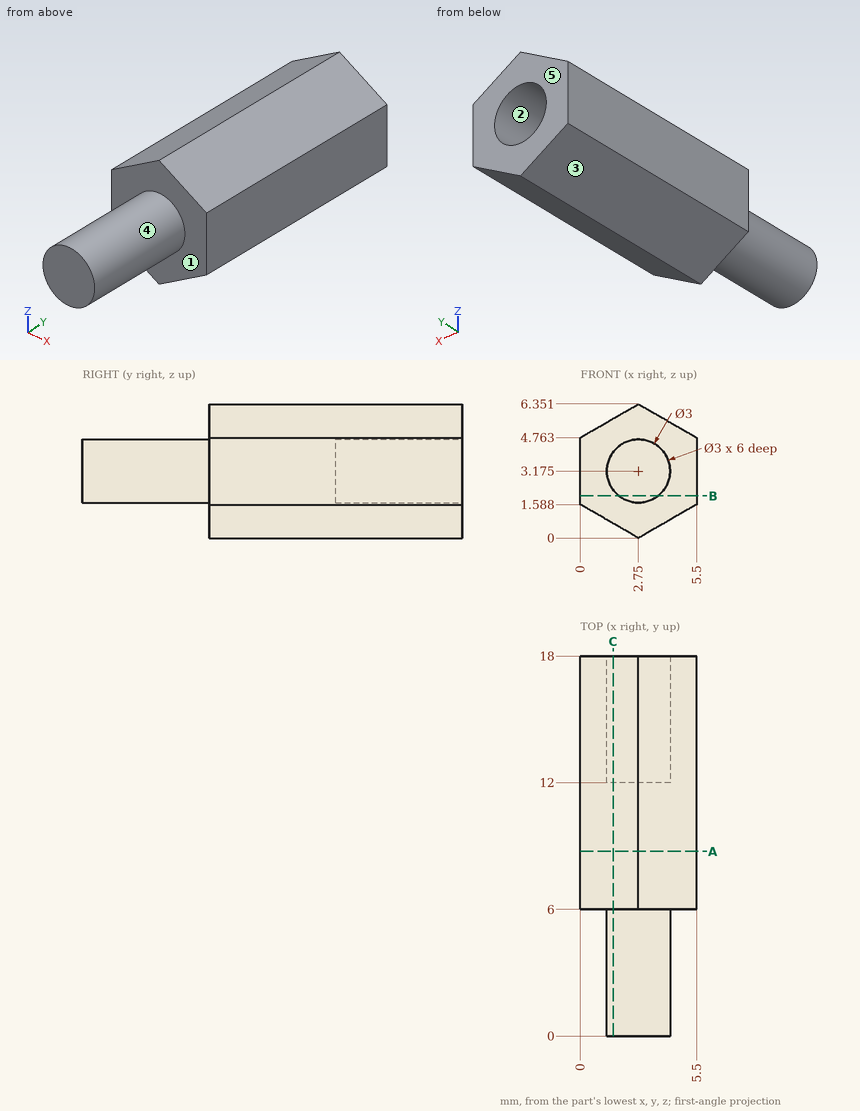
Print and shaded views of the part. All mm, measured from the part's lowest x, y and z. A direction names the side the tool comes from. Round coordinates to 2 decimals unless told otherwise and drop trailing zeros. Write each loop counter-clockwise with the first axis right and the second up, starting at its lowest first coordinate (ties: lowest second). Pieces come first, ordered by that corner, then holes. Notation, with made-up numbers: M 61.5,-27.5 L 74.5,-27.5 A26 cw 74.5,-2.5 Z; hole C -5.75,-28.75 d3. An arc over 180 degrees is marked long. One line per question, with ' | ' between items.
(1) Probe line 1 along Y through (x, z) = (0.5, 3.5); line 2 along Z through (x, y) = (2, 14.5) (1 decimal); line 3 along X through (y, z) = (16, 2.75). List the from-to ranges inside material, lowest first.
Answer key:
line 1: y = 6 to 18 | line 2: z = 0.4 to 1.9, 4.5 to 5.9 | line 3: x = 0 to 1.31, 4.19 to 5.5
(2) 3-axis set-ups, long thin cutter, end or side, ignore diameter. For the marked faces 4 and 5: which of +Z, -Z, +X, -X, +Y, -Y reach the whole face in a straight line?
Answer key:
face 4: -Y | face 5: +Z, -Z, +X, -X, +Y
(3) Saw through at A-A on y = 8.75. Write the cut outline in (x, z), then the cut area to 3 significant figures.
Answer key:
outline: M 0,1.59 L 2.75,0 L 5.5,1.59 L 5.5,4.76 L 2.75,6.35 L 0,4.76 Z | area: 26.2 mm^2
(4) Two-plate mould, pull along X, no slides. Class the marked faces 1, 2 and 3: released by +X, released by -X, zero draft, split by the parting line, or undercut.
Answer key:
face 1: zero draft | face 2: undercut | face 3: released by -X
(5) Saw through at B-B on z = 2. Write the cut outline in (x, y).
Answer key:
outline: M 0,6 L 1.82,6 L 1.82,0 L 3.68,0 L 3.68,6 L 5.5,6 L 5.5,18 L 3.68,18 L 3.68,12 L 1.82,12 L 1.82,18 L 0,18 Z
(6) Pin check, flat tip, straight feed: pin 1 (2 mm diameter, centred on x = 1.5, y = 8.5, fed in from +Z). Stop position of the tip, or through.
Answer key:
pin 1: stops at z = 6.21
(7) Saw through at C-C on x = 1.55. Write the cut outline in (y, z) (1 decimal).
Answer key:
outline: M 0,2.3 L 6,2.3 L 6,0.7 L 18,0.7 L 18,2.3 L 12,2.3 L 12,4.1 L 18,4.1 L 18,5.7 L 6,5.7 L 6,4.1 L 0,4.1 Z
